Source: CAD feature listing. Evaluate the final solid. Frame: model axes, mm. A direction names the side the tool comes from. Give positions to 0.01 mm unless a question says otherwise; leave off trailing zeros. Answer as CSV lines item,"result".
```python
from build123d import *

# Parameters (mm, degrees)
F0_R     = 158.75
F0_R_2   = 4.7625
F1_DEPTH = 50.8
F2_R     = 12.7


with BuildPart() as f1:
    # F0 (on Front) → F1 (new body)
    with BuildSketch(Plane.XZ):
        with Locations((-53.951404, 5.726499)):
            Circle(F0_R)
        with BuildLine():
            Line((-122.349605, -69.769714), (-71.433156, -18.853265))
            ThreePointArc((-71.433156, -18.853265), (-66.435836, -21.731021), (-60.982177, -23.605133))
            Line((-60.982177, -23.605133), (-60.982177, -95.783764))
            Line((-60.982177, -95.783764), (-60.982177, -101.994301))
            ThreePointArc((-60.982177, -101.994301), (-96.191027, -93.616427), (-126.652027, -74.072136))
            Line((-126.652027, -74.072136), (-122.349605, -69.769714))
        make_face(mode=Mode.SUBTRACT)
        with BuildLine():
            Line((-155.70012, 0.707446), (-83.693387, 0.707446))
            ThreePointArc((-83.693387, 0.707446), (-82.194629, -4.861074), (-79.663508, -10.04259))
            Line((-79.663508, -10.04259), (-130.701507, -61.080589))
            Line((-130.701507, -61.080589), (-135.09302, -65.472102))
            ThreePointArc((-135.09302, -65.472102), (-154.065384, -34.651634), (-161.784663, 0.707446))
            Line((-161.784663, 0.707446), (-155.70012, 0.707446))
        make_face(mode=Mode.SUBTRACT)
        with BuildLine():
            Line((-48.932352, -96.022217), (-48.932352, -24.015484))
            ThreePointArc((-48.932352, -24.015484), (-43.363832, -22.516726), (-38.182316, -19.985605))
            Line((-38.182316, -19.985605), (12.855683, -71.023604))
            Line((12.855683, -71.023604), (17.247196, -75.415117))
            ThreePointArc((17.247196, -75.415117), (-13.573272, -94.387481), (-48.932352, -102.10676))
            Line((-48.932352, -102.10676), (-48.932352, -96.022217))
        make_face(mode=Mode.SUBTRACT)
        with BuildLine():
            Line((21.544808, -62.671702), (-29.371641, -11.755253))
            ThreePointArc((-29.371641, -11.755253), (-26.493885, -6.757933), (-24.619772, -1.304274))
            Line((-24.619772, -1.304274), (47.558858, -1.304274))
            Line((47.558858, -1.304274), (53.769395, -1.304274))
            ThreePointArc((53.769395, -1.304274), (45.391521, -36.513124), (25.84723, -66.974124))
            Line((25.84723, -66.974124), (21.544808, -62.671702))
        make_face(mode=Mode.SUBTRACT)
        with BuildLine():
            ThreePointArc((-78.531168, 23.20825), (-81.408924, 18.21093), (-83.283036, 12.757272))
            Line((-83.283036, 12.757272), (-155.461667, 12.757272))
            Line((-155.461667, 12.757272), (-161.672204, 12.757272))
            ThreePointArc((-161.672204, 12.757272), (-153.29433, 47.966121), (-133.750039, 78.427121))
            Line((-133.750039, 78.427121), (-129.447617, 74.124699))
            Line((-129.447617, 74.124699), (-78.531168, 23.20825))
        make_face(mode=Mode.SUBTRACT)
        with BuildLine():
            ThreePointArc((-125.150005, 86.868114), (-94.329537, 105.840478), (-58.970457, 113.559757))
            Line((-58.970457, 113.559757), (-58.970457, 107.475214))
            Line((-58.970457, 107.475214), (-58.970457, 35.468481))
            ThreePointArc((-58.970457, 35.468481), (-64.538977, 33.969723), (-69.720493, 31.438602))
            Line((-69.720493, 31.438602), (-120.758492, 82.476601))
            Line((-120.758492, 82.476601), (-125.150005, 86.868114))
        make_face(mode=Mode.SUBTRACT)
        with Locations((-53.951404, 5.726499)):
            Circle(F0_R_2, mode=Mode.SUBTRACT)
        with BuildLine():
            ThreePointArc((-24.209422, 10.745551), (-25.70818, 16.314071), (-28.239301, 21.495587))
            Line((-28.239301, 21.495587), (22.798698, 72.533586))
            Line((22.798698, 72.533586), (27.190211, 76.925099))
            ThreePointArc((27.190211, 76.925099), (46.162575, 46.104631), (53.881854, 10.745551))
            Line((53.881854, 10.745551), (47.797311, 10.745551))
            Line((47.797311, 10.745551), (-24.209422, 10.745551))
        make_face(mode=Mode.SUBTRACT)
        with BuildLine():
            Line((14.446796, 81.222711), (-36.469653, 30.306262))
            ThreePointArc((-36.469653, 30.306262), (-41.466973, 33.184018), (-46.920631, 35.058131))
            Line((-46.920631, 35.058131), (-46.920631, 107.236761))
            Line((-46.920631, 107.236761), (-46.920631, 113.447298))
            ThreePointArc((-46.920631, 113.447298), (-11.711782, 105.069424), (18.749218, 85.525133))
            Line((18.749218, 85.525133), (14.446796, 81.222711))
        make_face(mode=Mode.SUBTRACT)
    extrude(amount=F1_DEPTH)

    # F2
    f2_edges = [f1.edges().sort_by_distance(p)[0] for p in [
        (-212.701404, -50.8, 5.726499),
        (-212.701404, 0, 5.726499),
    ]]
    fillet(f2_edges, radius=F2_R)


solid = f1.part
```
(1) Contact query for flat-ended pins moving along their axis: pin 1 (12 mm diameter, centred on y = -7.5, z = -25, fed in from -X); pin 2 (15 mm diameter, centred on y = -19, z = 87, fed in from +X); pin 3 (5 mm diameter, centred on x = -98, y = -42, fed in from +Z). Output: stop coordinate, or through.
Completed:
pin 1,"x = -210.47"
pin 2,"x = 86.62"
pin 3,"z = 158.57"
(2) Cut plane A-A (y = -43). Give the number of separate pieces and of enclosed holes in the cut face, then the cut area to 3 significant figures.
Completed:
separate pieces,"1"
enclosed holes,"9"
area,"51,900 mm²"
(3) Access query for faces 4 (the flat face through (-24, 0, 8)), 5 (the flat face through (-106.99, -25.04, -37.37)). Directions: +Z, -Z, +X, -X, +Y, -Y. A direction counts if a zero-diameter tool reaches every point of the face in a straight line with its end or side. Return the directions, or none.
Completed:
face 4,"+Z, -Z, +X, -X, +Y"
face 5,"+Y, -Y"
(4) Mould query, pull axis X, two halves, no side actions, for faces 1 (the cylindrical face through (-64.46, -25.04, 34)), 2 (the flat face through (-24, -50.8, 8)), 3 (the flat face through (-123, -25, 0.707)). Classes: released by +X, released by -X, zero draft, split by the parting line, or undercut.
Completed:
face 1,"undercut"
face 2,"zero draft"
face 3,"undercut"
(5) Ray query, line 1 (Z direction, x = 34.5, y = -43); line 2 (Z direction, x = -74.5, y = -4); line 3 (X direction, y = -31.5, z = 37.5). Return the intervals inside material, ascending. Write a range as from..to.
Completed:
line 1,"-124.91..-56.16, -1.3..10.75, 67.61..136.37"
line 2,"-148.21..-100.25, -21.92..36.22, 111.7..159.66"
line 3,"-209.49..-157.12, -92.82..-75.78, -58.97..-46.92, -29.28..-12.23, 49.22..101.59"
